The model under review builds one solid part; all positions refer to its coordinate system, in mm. A direction names the side the tool comes from. Coordinates: 2 decimals unless noted, no trailing zeros. Write each loop counter-clockwise with the first axis right and the second up, starting at its lowest first coordinate (ties: lowest second). Pieces come first, ordered by that corner, then holes. Notation, with made-up numbers: M -27,-36.5 L 3,-36.5 A28 ccw 3,-1.5 Z; hole C -31.75,32.5 d7. An arc over 180 degrees is marked long. Answer as a JSON object with one key per item and string values.
```python
from build123d import *

# Parameters (mm, degrees)
EXTRUDE1_START = 7.399
SKETCH2_R      = 5.4125
EXTRUDE1_DEPTH = 7.399


with BuildPart() as part:
    # Sketch1 → Revolve1 (revolve)
    with BuildSketch(Plane.XY, mode=Mode.PRIVATE) as revolve1_sk:
        Polygon((0, 4.7625), (0, 8.3185), (0.4445, 8.763), (0.889, 8.763), (0.889, 5.4125), (18.288, 5.4125), (18.288, 4.7625), align=None)
    revolve(revolve1_sk.sketch.rotate(Axis((0, 0, 0), (1, 0, 0)), 90), axis=Axis((0, 0, 0), (1, 0, 0)))

    # Sketch2 → Extrude1 (add)
    with BuildSketch(Plane(origin=(0.889, 0, 0), x_dir=(0, 0, -1), z_dir=(1, 0, 0)).offset(EXTRUDE1_START)):
        Polygon((7.332348419, 0), (3.666174209, 6.35), (-3.666174209, 6.35), (-7.332348419, 0), (-3.666174209, -6.35), (3.666174209, -6.35), align=None)
        with Locations(Location((0, 0, 0), (0, 0, 180))):
            Circle(SKETCH2_R, mode=Mode.SUBTRACT)
    extrude(amount=-EXTRUDE1_DEPTH)


solid = part.part
```
(1) For pin 1 Ø3 at (x, y) = (10, -6) entering from -Z; pin 2 Ø3.5 at (x, z) = (3, -1.5) entering from +Y; pin 3 Ø8 at (x, z) = (5, 1.5) entering from -Y, all flat-tipped, find the tip position at first contact; note any pin that passes through.
Results list:
{"pin 1": "z = -3.01", "pin 2": "y = 6.35", "pin 3": "y = -6.35"}
(2) Draft analysis for pull direction Z (two halves, no side actions). For faces 1 (the face through (5, -6.35, 0)), 2 (the face through (4.64, -3.131, 5.525)), 3 (the face through (9.02, 4.65, -1.03)), 4 (the face through (4.64, -3.219, -5.474)), state which applies: released by +Z, released by -Z, zero draft, split by the parting line, or undercut.
Results list:
{"face 1": "zero draft", "face 2": "released by +Z", "face 3": "undercut", "face 4": "released by -Z"}
(3) Wall thickness on line 1 along Y through (x, z) = (6.5, 0); line 2 along Y through (x, z) = (12, 0); line 3 along Z through (x, y) = (14, 3.75): over which ranges is each line inside the solid? List them lowest first. Write a range as from..to.
Results list:
{"line 1": "-6.35..-4.76, 4.76..6.35", "line 2": "-5.41..-4.76, 4.76..5.41", "line 3": "-3.9..-2.94, 2.94..3.9"}
(4) Add section C-C on x = 11. Give the boundary of the cut face in (y, z) (1 decimal).
Results list:
{"outline": "C 0,0 d10.8; hole C 0,0 d9.5"}
(5) Add section A-A on z = 0. Give the boundary of the cut face in (x, y), and give its area (3 significant figures).
Results list:
{"outline": "M 0,-8.32 L 0.44,-8.76 L 0.89,-8.76 L 0.89,-6.35 L 8.29,-6.35 L 8.29,-5.41 L 18.29,-5.41 L 18.29,-4.76 L 0,-4.76 Z; M 0,4.76 L 18.29,4.76 L 18.29,5.41 L 8.29,5.41 L 8.29,6.35 L 0.89,6.35 L 0.89,8.76 L 0.44,8.76 L 0,8.32 Z", "area": "43.4 mm²"}
(6) For faces 5 (the face through (8.288, -1.4, -5.4)), 6 (the face through (4.64, 3.219, 5.474)), 7 (the face through (4.64, 3.131, -5.525)), list the 3-axis set-ups (+Z, -Z, +X, -X, +Y, -Y) from which the entire face can be reached by the end or side of a thin tool; tool diameter is ignored.
Results list:
{"face 5": "+X", "face 6": "+Z, +X, +Y", "face 7": "-Z, +X, +Y"}
